from build123d import *

# Parameters (mm, degrees)
SKETCH_R     = 7.5
PAD_DEPTH    = 9
SKETCH001_R  = 7.5
PAD001_DEPTH = 2
SKETCH002_R  = 7.5
PAD002_DEPTH = 9
SKETCH003_R  = 7.5
PAD003_DEPTH = 1.5
SKETCH004_R  = 7.5
PAD004_DEPTH = 5.5
PAD005_DEPTH = 21.5
SKETCH006_R  = 12.5
PAD006_DEPTH = 5
SKETCH007_W  = 35.462824
SKETCH007_H  = 56.081524
SKETCH007_R  = 2.5
PAD007_DEPTH = 5


with BuildPart() as part:
    # Sketch → Pad (new body)
    with BuildSketch(Plane.XY):
        Circle(SKETCH_R)
    extrude(amount=PAD_DEPTH)

    # Sketch001 (on Face3 of Pad) → Pad001 (join)
    with BuildSketch(Plane.XY.offset(9)):
        Circle(SKETCH001_R)
    extrude(amount=PAD001_DEPTH)

    # Sketch002 (on Face4 of Pad001) → Pad002 (join)
    with BuildSketch(Plane.XY.offset(11)):
        Circle(SKETCH002_R)
    extrude(amount=PAD002_DEPTH)

    # Sketch003 (on Face5 of Pad002) → Pad003 (join)
    with BuildSketch(Plane.XY.offset(20)):
        Circle(SKETCH003_R)
    extrude(amount=PAD003_DEPTH)

    # Sketch004 (on Face2 of Pad003) → Pad004 (join)
    with BuildSketch(Plane(origin=(0, 0, 0), x_dir=(1, 0, 0), z_dir=(0, 0, -1))):
        Circle(SKETCH004_R)
    extrude(amount=PAD004_DEPTH)

    # Sketch005 (on Face4 of Pad004) → Pad005 (join)
    with BuildSketch(Plane(origin=(0, 0, -5.5), x_dir=(1, 0, 0), z_dir=(0, 0, -1))):
        with BuildLine():
            Line((3.5, 2), (3.5, -2))
            Line((3.5, -2), (7.228416, -2))
            ThreePointArc((7.228416, -2), (7.5, 0), (7.228416, 2))
            Line((3.5, 2), (7.228416, 2))
        make_face()
        with BuildLine():
            Line((-3.5, 2), (-3.5, -2))
            Line((-3.5, -2), (-7.228416, -2))
            ThreePointArc((-7.228416, 2), (-7.5, 0), (-7.228416, -2))
            Line((-3.5, 2), (-7.228416, 2))
        make_face()
    extrude(amount=PAD005_DEPTH)

    # Sketch006 (on Face15 of Pad005) → Pad006 (join)
    with BuildSketch(Plane(origin=(0, 0, -27), x_dir=(1, 0, 0), z_dir=(0, 0, -1))):
        Circle(SKETCH006_R)
        with BuildLine():
            ThreePointArc((10.816654, 2), (0, 11), (-10.816654, 2))
            Line((-3.5, 2), (-10.816654, 2))
            Line((-3.5, -2), (-3.5, 2))
            Line((-10.816654, -2), (-3.5, -2))
            ThreePointArc((-10.816654, -2), (0, -11), (10.816654, -2))
            Line((10.816654, -2), (3.5, -2))
            Line((3.5, -2), (3.5, 2))
            Line((3.5, 2), (10.816654, 2))
        make_face(mode=Mode.SUBTRACT)
    extrude(amount=-PAD006_DEPTH)

    # Sketch007 (on Face31 of Pad006) → Pad007 (join)
    with BuildSketch(Plane(origin=(0, 0, -27), x_dir=(1, 0, 0), z_dir=(0, 0, -1))):
        with Locations((0, 3.914595)):
            Rectangle(SKETCH007_W, SKETCH007_H)
        with Locations((0, 25)):
            Circle(SKETCH007_R, mode=Mode.SUBTRACT)
        with Locations((0, -15)):
            Circle(SKETCH007_R, mode=Mode.SUBTRACT)
        Circle(SKETCH007_R, mode=Mode.SUBTRACT)
    extrude(amount=-PAD007_DEPTH)


solid = part.part
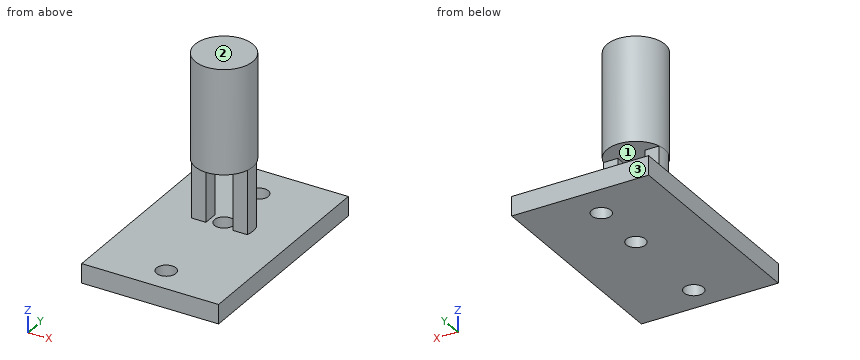
Part model, mm, in its own coordinate system. Face numbers are marked on the shaded views. Give positions to 0.01 mm unless a question says otherwise; leave off trailing zeros. Loops run counter-clockwise (first coordinate to the right, second up) from the corner with the lowest first, then second, coordinate; pieces in that order, holes last. Notation, with made-up numbers: (20, -26.5) -> (30, -26.5) arc R6 ccw to (30, -21.5) -> close; hole circle Ø3 at (15, 3.5). An arc over 180 degrees is marked (long way). Write each question's results on one line, items separated by ' | '. Start each with the question number.
Q1. Band-saw the part on B-B on x = 0. List the corners of the cut face in (y, z), plus the area to 3 significant figures.
Q2. Band-saw the part on A-A on y = -25. List the corners of the cut face in (x, z).
Q3. Band-saw the part on D-D on x = -9. List the corners of the cut face in (y, z), plus the area to 3 significant figures.
Q4. Band-saw the part on C-C on y = 0. List the corners of the cut face in (x, z).
Q5. Pull direction Z, two halves, no side cores. Call the marked faces 1, 2 and 3: +Z half, -Z half, draft (parallel to the pull), parting line (faces both ways), or undercut.
Q6. Pin check, flat tips, straight feed: P1, Ø8, axis at x = -7.5, z = 2, coming from the -Y side; P2, Ø2, axis at y = 4.5, z = 10.5, coming from the +X side; P3, Ø6.5, axis at x = 0, y = 15, coming from the -Z side; P4, Ø8, axis at x = 2.5, y = -23, coming from the +Z side. Stop position of each tip, or through.
Q7. Wall check: L1, parallel to X at y = 15, z = -25; L2, parallel to Y at x = 0, z = -23; L3, parallel to Z at x = 3, y = 5. Give the ranges that are in metal, low to high.
Results are:
1) outline: (-31.96, -27) -> (-27.5, -27) -> (-27.5, -22) -> (-31.96, -22) -> close; (-22.5, -27) -> (-2.5, -27) -> (-2.5, -22) -> (-22.5, -22) -> close; (-7.5, -5.5) -> (7.5, -5.5) -> (7.5, 21.5) -> (-7.5, 21.5) -> close; (2.5, -27) -> (12.5, -27) -> (12.5, -22) -> (2.5, -22) -> close; (17.5, -27) -> (24.13, -27) -> (24.13, -22) -> (17.5, -22) -> close | area: 610 mm²
2) outline: (-17.73, -27) -> (-2.5, -27) -> (-2.5, -22) -> (-17.73, -22) -> close; (2.5, -27) -> (17.73, -27) -> (17.73, -22) -> (2.5, -22) -> close
3) outline: (-31.96, -27) -> (24.13, -27) -> (24.13, -22) -> (-31.96, -22) -> close | area: 280 mm²
4) outline: (-17.73, -27) -> (-2.5, -27) -> (-2.5, -22) -> (-3.5, -22) -> (-3.5, -5.5) -> (3.5, -5.5) -> (3.5, -22) -> (2.5, -22) -> (2.5, -27) -> (17.73, -27) -> (17.73, -22) -> (7.5, -22) -> (7.5, 21.5) -> (-7.5, 21.5) -> (-7.5, -22) -> (-17.73, -22) -> close
5) face 1: undercut | face 2: +Z half | face 3: draft
6) P1: stops at y = -6.63 | P2: stops at x = 6.63 | P3: stops at z = -27 | P4: stops at z = -22
7) L1: x = -17.73 to -2.5, 2.5 to 17.73 | L2: y = -31.96 to -27.5, -22.5 to -2.5, 2.5 to 12.5, 17.5 to 24.13 | L3: z = -27 to -22, -5.5 to 21.5
